The model under review builds one solid part; all positions refer to its coordinate system, in mm. A direction names the side the tool comes from. Give positions to 0.01 mm unless a question says otherwise; leave off trailing zeros. Order: outer loops, then holes, each group sorted by start corner. A loop starts at its lowest first (then second) coordinate and runs counter-clockwise, first axis right, second up. Notation, with made-up numbers: (2.5, -37) - (57.5, -37) arc R20 ccw to (57.5, 2) - close; hole circle Ø6 at (15, 41). An arc over 180 degrees is marked (long way). Use CSV: the item, a comma, the result in double quotes.
```python
from build123d import *

# Parameters (mm, degrees)
BOSS_EXTRUDE1_DEPTH = 2


with BuildPart() as part:
    # Model → Boss-Extrude1 (new body)
    with BuildSketch(Plane.XY):
        with BuildLine():
            Line((1971.609841287, 1160.893641222), (1971.609841287, 1159.893641222))
            ThreePointArc((1971.609841287, 1159.893641222), (1972.609841287, 1157.893641222), (1973.609841287, 1159.893641222))
            Line((1973.609841287, 1159.893641222), (1973.609841287, 1160.893641222))
            Line((1973.609841287, 1160.893641222), (1976.609841287, 1160.893641222))
            Line((1976.609841287, 1160.893641222), (1976.609841287, 1159.893641222))
            ThreePointArc((1976.609841287, 1159.893641222), (1977.609841287, 1157.893641222), (1978.609841287, 1159.893641222))
            Line((1978.609841287, 1159.893641222), (1978.609841287, 1160.893641222))
            Line((1978.609841287, 1160.893641222), (1979.859841287, 1160.893641222))
            ThreePointArc((1979.859841287, 1160.893641222), (1980.566948068, 1160.600748003), (1980.859841287, 1159.893641222))
            Line((1980.859841287, 1159.893641222), (1980.859841287, 1156.893641222))
            Line((1980.859841287, 1156.893641222), (1979.609841287, 1156.893641222))
            Line((1979.609841287, 1156.893641222), (1979.609841287, 1154.893641222))
            Line((1979.609841287, 1154.893641222), (1970.609841287, 1154.893641222))
            Line((1970.609841287, 1154.893641222), (1970.609841287, 1156.893641222))
            Line((1970.609841287, 1156.893641222), (1969.359841287, 1156.893641222))
            Line((1969.359841287, 1156.893641222), (1969.359841287, 1159.893641222))
            ThreePointArc((1969.359841287, 1159.893641222), (1969.652734505, 1160.600748003), (1970.359841287, 1160.893641222))
            Line((1970.359841287, 1160.893641222), (1971.609841287, 1160.893641222))
        make_face()
    extrude(amount=BOSS_EXTRUDE1_DEPTH)


solid = part.part
```
Item 1: Wall thickness on L1, parallel to X at y = 1159.15, z = 1.2; L2, parallel to X at y = 1158.1, z = 0.1; L3, parallel to X at y = 1155.4, z = 1.4: over which ranges is each line inside the solid? List them lowest first.
Results list:
L1,"x = 1969.36 to 1971.36, 1973.86 to 1976.36, 1978.86 to 1980.86"
L2,"x = 1969.36 to 1971.92, 1973.3 to 1976.92, 1978.3 to 1980.86"
L3,"x = 1970.61 to 1979.61"
Item 2: Take a section at C-C, the plane y = 1155.6. Give the boundary of the cut face in (x, z), and give its area (3 significant figures).
Results list:
outline,"(1970.61, 0) - (1979.61, 0) - (1979.61, 2) - (1970.61, 2) - close"
area,"18.0 mm2"
Item 3: Take a section at D-D, the plane x = 1970.25. Give the boundary of the cut face in (y, z), and give its area (3 significant figures).
Results list:
outline,"(1156.89, 0) - (1160.89, 0) - (1160.89, 2) - (1156.89, 2) - close"
area,"7.99 mm2"
Item 4: Take a section at B-B, the plane y = 1160.4. Give the boundary of the cut face in (x, z), and give its area (3 significant figures).
Results list:
outline,"(1969.5, 0) - (1971.61, 0) - (1971.61, 2) - (1969.5, 2) - close; (1973.61, 0) - (1976.61, 0) - (1976.61, 2) - (1973.61, 2) - close; (1978.61, 0) - (1980.72, 0) - (1980.72, 2) - (1978.61, 2) - close"
area,"14.4 mm2"
Item 5: Mouldability with a two-part tool opening along Y and no side actions: class faces 1 (the face through (1972.571, 1157.894, 0.986)), 2 (the face through (1978.61, 1160.4, 1)), 3 (the face through (1975, 1154.894, 1)) as pulls with the +Y half, pulls with the -Y half, needs draft (parallel to the pull), parting line crosses it, or undercut.
Results list:
face 1,"undercut"
face 2,"needs draft"
face 3,"pulls with the -Y half"
Item 6: Clearance check with flat-ended pins moving along their axes: pin 1 (0.6 mm diameter, centred on x = 1980, z = 1.5, fed in from -Y); pin 2 (0.5 mm diameter, centred on y = 1160.5, z = 1.5, fed in from -X); pin 3 (1 mm diameter, centred on y = 1156, z = 0.5, fed in from +X). State where each tip first meets the part, or that it passes through.
Results list:
pin 1,"stops at y = 1156.89"
pin 2,"stops at x = 1969.43"
pin 3,"stops at x = 1979.61"
Item 7: Tool access review of faces 4 (the face through (1970.61, 1156, 1)), 5 (the face through (1971.61, 1160.4, 1)), 6 (the face through (1979.61, 1156, 1)), 7 (the face through (1977.571, 1157.894, 0.986)), 8 (the face through (1980.86, 1158, 1)): name each direction out of +Z, -Z, +X, -X, +Y, -Y from which nothing blocks a thin tool from reaching the whole face with its end or side.
Results list:
face 4,"+Z, -Z, -X, -Y"
face 5,"+Z, -Z, +Y"
face 6,"+Z, -Z, +X, -Y"
face 7,"+Z, -Z"
face 8,"+Z, -Z, +X, +Y, -Y"
Item 8: Take a section at A-A, the plane z = 1.45. Give the boundary of the cut face in (x, y), and give its area (3 significant figures).
Results list:
outline,"(1969.36, 1156.89) - (1970.61, 1156.89) - (1970.61, 1154.89) - (1979.61, 1154.89) - (1979.61, 1156.89) - (1980.86, 1156.89) - (1980.86, 1159.89) arc R1 ccw to (1979.86, 1160.89) - (1978.61, 1160.89) - (1978.61, 1159.89) arc R1.25 cw (long way) to (1976.61, 1159.89) - (1976.61, 1160.89) - (1973.61, 1160.89) - (1973.61, 1159.89) arc R1.25 cw (long way) to (1971.61, 1159.89) - (1971.61, 1160.89) - (1970.36, 1160.89) arc R1 ccw to (1969.36, 1159.89) - close"
area,"51.2 mm2"
